from build123d import *

# Parameters (mm, degrees)
F1_W     = 107.696
F1_H     = 107.696
F1_W_2   = 101.6
F1_H_2   = 101.6
F2_DEPTH = 3.81
F0_W     = 101.6
F0_H     = 101.6
F3_DEPTH = 3.302
F4_DEPTH = 5.08


with BuildPart() as f2:
    # F1 (on face) → F2 (new body)
    with BuildSketch(Plane.XY):
        Rectangle(F1_W, F1_H)
        Rectangle(F1_W_2, F1_H_2, mode=Mode.SUBTRACT)
    extrude(amount=F2_DEPTH)

    # F0 (on Top) → F3 (join)
    with BuildSketch(Plane.XY):
        Rectangle(F0_W, F0_H)
    extrude(amount=F3_DEPTH)

    # F4 (add): a face of the model
    f4_faces = [f2.faces().sort_by_distance(p)[0] for p in [
        (-52.3249485619, 0, 3.81),
    ]]
    extrude(f4_faces, amount=F4_DEPTH)


solid = f2.part
Check sheet for the modelled part. Datum: model origin and axes. Units: mm. A direction names the side the tool comes from. Give positions to 0.01 mm unless a question says otherwise; leave off trailing zeros. Write each loop counter-clockwise with the first axis right and the second up, starting at its lowest first coordinate (ties: lowest second). Pieces come first, ordered by that corner, then holes. Notation, with made-up numbers: (74, 27) -> (123, 27) arc R6 cw to (123, 35) -> close; hole circle Ø2 at (-0.75, 65.25). An arc over 180 degrees is marked (long way). Use one line per item in the form item = value. Start each with the question number.
1. Go/stop test with a flat-tipped pin: P1, Ø10, axis at x = 0, y = -16.5, coming from the +Z side. Record where the tip stops, or that it passes through.
2. Section check B-B (x = -25.5). Record the cut outline in (y, z), and give its area (3 significant figures).
3. Access from +Z, -Z, +X, -X, +Y, -Y to the whole of each face (thin tool, end or side, straight path). Record for faces 1 (the flat face through (53.848, -1, 4)), 2 (the flat face through (50.8, -1, 6)).
4. Thickness scan on line 1 along Y through (x, z) = (-41, 5.25); line 2 along Z through (x, y) = (30.5, -24). Record the ranges inside material, lowest first. Write a range as from..to.
5. Mould release check, pull along X, two halves, no side actions. Record for faces 3 (the flat face through (-1, 50.8, 6)), 4 (the flat face through (-1, 1, 0)), 5 (the flat face through (-53.848, -1, 4)): pulls with the +X half, pulls with the -X half, needs draft (parallel to the pull), parting line crosses it, or undercut.
6. Section check A-A (z = 7.25). Record the cut outline in (x, y), and give its area (3 significant figures).
Conclusion:
q1.P1 = 3.3
q2.outline = (-53.85, 0) -> (53.85, 0) -> (53.85, 8.89) -> (50.8, 8.89) -> (50.8, 3.3) -> (-50.8, 3.3) -> (-50.8, 8.89) -> (-53.85, 8.89) -> close
q2.area = 390 mm²
q3.face_1 = +Z, -Z, +X, +Y, -Y
q3.face_2 = +Z
q4.line_1 = -53.85..-50.8, 50.8..53.85
q4.line_2 = 0..3.3
q5.face_3 = undercut
q5.face_4 = needs draft
q5.face_5 = pulls with the -X half
q6.outline = (-53.85, -53.85) -> (53.85, -53.85) -> (53.85, 53.85) -> (-53.85, 53.85) -> close; hole (-50.8, -50.8) -> (50.8, -50.8) -> (50.8, 50.8) -> (-50.8, 50.8) -> close
q6.area = 1,280 mm²
